from build123d import *

# Parameters (mm, degrees)
F0_R     = 69.85
F1_DEPTH = 6.35
F2_R     = 12.7
F3_R     = 3.175
F4_DEPTH = 6.35
F6_DEPTH = 6.35


with BuildPart() as f1:
    # F0 (on Top) → F1 (new body)
    with BuildSketch(Plane.XY):
        Polygon((64.5896307397, 88.9), (-64.5896307397, 88.9), (-104.5082178576, -33.9567784001), (0, -109.8864431997), (104.5082178576, -33.9567784001), align=None)
        Circle(F0_R, mode=Mode.SUBTRACT)
    extrude(amount=F1_DEPTH)

    # F2
    f2_edges = [f1.edges().sort_by_distance(p)[0] for p in [
        (-64.589631, 88.9, 3.175),
        (-104.508218, -33.956778, 3.175),
        (0, -109.886443, 3.175),
        (104.508218, -33.956778, 3.175),
        (64.589631, 88.9, 3.175),
    ]]
    fillet(f2_edges, radius=F2_R)

    # F3 (on face) → F4 (cut, through all)
    with BuildSketch(Plane.XY.offset(6.35)):
        with Locations((0, -98.425)):
            Circle(F3_R)
        with Locations((93.6077376164, -30.4149976714)):
            Circle(F3_R)
        with Locations((57.8527634569, 79.6274976714)):
            Circle(F3_R)
        with Locations((-57.8527634569, 79.6274976714)):
            Circle(F3_R)
        with Locations((-93.6077376164, -30.4149976714)):
            Circle(F3_R)
    extrude(amount=-F4_DEPTH, mode=Mode.SUBTRACT)

    # F5 (on face) → F6 (cut, through all)
    with BuildSketch(Plane.XY.offset(6.35)):
        with BuildLine():
            Line((55.362540634, 88.9), (-55.362540634, 88.9))
            ThreePointArc((-55.362540634, 88.9), (0, 84.5639308192), (55.362540634, 88.9))
        make_face()
        with BuildLine():
            ThreePointArc((-101.6568902063, -25.1812942287), (-80.4250774491, 26.1316917343), (-67.440958391, 80.1245158286))
            Line((-67.440958391, 80.1245158286), (-101.6568902063, -25.1812942287))
        make_face()
        with BuildLine():
            ThreePointArc((-7.4648727041, -104.462895714), (-49.7054314114, -68.4136571439), (-97.0433451535, -39.3803258858))
            Line((-97.0433451535, -39.3803258858), (-7.4648727041, -104.462895714))
        make_face()
        with BuildLine():
            ThreePointArc((97.0433451535, -39.3803258858), (49.7054314114, -68.4136571439), (7.4648727041, -104.462895714))
            Line((7.4648727041, -104.462895714), (97.0433451535, -39.3803258858))
        make_face()
        with BuildLine():
            ThreePointArc((67.440958391, 80.1245158286), (80.4250774491, 26.1316917343), (101.6568902063, -25.1812942287))
            Line((101.6568902063, -25.1812942287), (67.440958391, 80.1245158286))
        make_face()
    extrude(amount=-F6_DEPTH, mode=Mode.SUBTRACT)


solid = f1.part
Design review of the part built by this model. Coordinates are the model's own, in mm. Coordinates: 2 decimals unless noted, no trailing zeros. Order: outer loops, then holes, each group sorted by start corner. A loop starts at its lowest first (then second) coordinate and runs counter-clockwise, first axis right, second up. Notation, with made-up numbers: M -15,86 L -9,86 A19 cw -9,100 Z; hole C 59,38.5 d1. An arc over 180 degrees is marked long. Use a Markdown table: item, result.
(1) Wall thickness on probe 1 along Y at (x, z) = (-60, 2); probe 2 along Y at (x, z) = (-59, 3); probe 3 along Y at (x, z) = (48.5, 4.75): over which ranges is each line inside the solid? List them lowest first.
Worked answers:
| item | result |
|---|---|
| probe 1 | y = -61.21 to -35.76, 35.76 to 77.29, 81.97 to 88.02 |
| probe 2 | y = -61.88 to -37.39, 37.39 to 76.67, 82.59 to 88.37 |
| probe 3 | y = -69.29 to -50.27, 50.27 to 87.89 |
(2) For P1, Ø4, axis at x = 93.61, y = -30.41, coming from the +Z side; P2, Ø2, axis at x = 12.5, z = 5.5, coming from the -Y side; P3, Ø3, axis at x = -21.5, z = 2, coming from the -Y side; P4, Ø2, axis at x = -36.5, z = 2, coming from the +Y side, all flat-tipped, find the tip position at first contact; note any pin that passes through.
Worked answers:
| item | result |
|---|---|
| P1 | passes through |
| P2 | stops at y = -100.5 |
| P3 | stops at y = -92.54 |
| P4 | stops at y = 86.55 |
(3) Add section D-D (x = -82). Give the boundary of the cut face in (y, z).
Worked answers:
| item | result |
|---|---|
| outline | M -47.52,0 L 21.4,0 L 21.4,6.35 L -47.52,6.35 Z |
(4) Draft analysis for pull direction X (two halves, no side actions). For faces 1 (the cylindrical face through (90.436, -30.275, 3.219)), 2 (the flat face through (-38, -59, 0)), 3 (the cylindrical face through (-80.666, 25.392, 3.219)), state which applies: released by +X, released by -X, zero draft, split by the parting line, or undercut.
Worked answers:
| item | result |
|---|---|
| face 1 | undercut |
| face 2 | zero draft |
| face 3 | released by -X |
(5) Add section A-A (y = -14). Give the boundary of the cut face in (x, z).
Worked answers:
| item | result |
|---|---|
| outline | M -96.21,0 L -68.43,0 L -68.43,6.35 L -96.21,6.35 Z; M 68.43,0 L 96.21,0 L 96.21,6.35 L 68.43,6.35 Z |
(6) Add section B-B (x = 14). Give the boundary of the cut face in (y, z), then the cut area to 3 significant figures.
Worked answers:
| item | result |
|---|---|
| outline | M -98.1,0 L -68.43,0 L -68.43,6.35 L -98.1,6.35 Z; M 68.43,0 L 84.84,0 L 84.84,6.35 L 68.43,6.35 Z |
| area | 293 mm2 |
(7) Add section C-C (z = 5.25). Count the separate pieces of the cut face and the enclosed holes in it, then the cut area to 3 significant figures.
Worked answers:
| item | result |
|---|---|
| separate pieces | 1 |
| enclosed holes | 6 |
| area | 11,500 mm2 |
